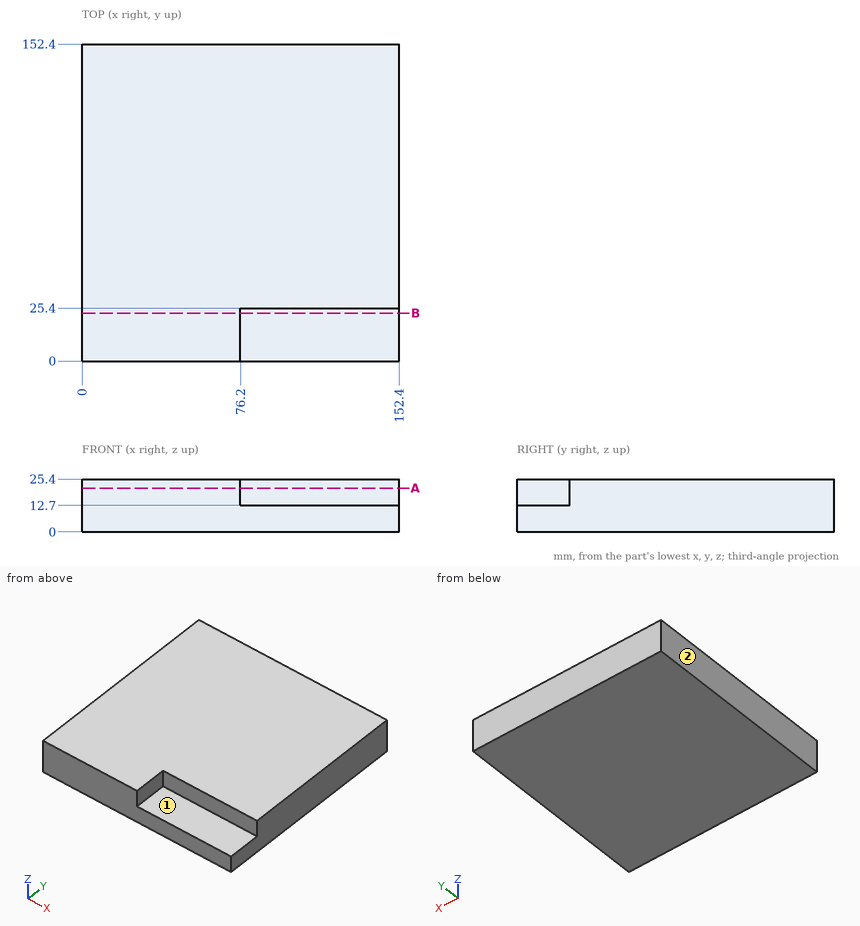
Design review of the part shown in the three views and the two pictorial views. Dimensions are in mm from the part's minimum x, y and z. A direction names the side the tool comes from. Coordinates: 2 decimals unless noted, no trailing zeros. Loops run counter-clockwise (first coordinate to the right, second up) from the corner with the lowest first, then second, coordinate; pieces in that order, holes last. Notation, with made-up numbers: M -24.75,43 L -6.75,43 A35 cw -6.75,80 Z; hole C 74.5,77 d11. An arc over 180 degrees is marked long. One line per question, with ' | ' between items.
(1) We need section B-B (y = 23). Give the boundary of the cut face in (x, z), and give its area (3 significant figures).
Filled in:
outline: M 0,0 L 152.4,0 L 152.4,12.7 L 76.2,12.7 L 76.2,25.4 L 0,25.4 Z | area: 2,900 mm^2
(2) For pin 1 Ø3 at (x, z) = (80.5, 17.5) entering from -Y, flat-tipped, find the tip position at first contact; note if it passes through.
Filled in:
pin 1: stops at y = 25.4
(3) Wall thickness on probe 1 along Y at (x, z) = (118, 21.5); probe 2 along Z at (x, y) = (97, 15.5): over which ranges is each line inside the solid? List them lowest first.
Filled in:
probe 1: y = 25.4 to 152.4 | probe 2: z = 0 to 12.7
(4) Machinability: for the marked faces 1 and 2, which of the approach directions +Z, -Z, +X, -X, +Y, -Y give a long, thin tool a straight path to every point of the face, cutting with its end or side? Answer none if there is none.
Filled in:
face 1: +Z, +X, -Y | face 2: +Z, -Z, -X, +Y, -Y
(5) We need section A-A (z = 21). Give the boundary of the cut face in (x, y), and give its area (3 significant figures).
Filled in:
outline: M 0,0 L 76.2,0 L 76.2,25.4 L 152.4,25.4 L 152.4,152.4 L 0,152.4 Z | area: 21,300 mm^2
